For this review, take the finished solid that the model builds, in its own axes (mm). Round coordinates to 2 decimals unless told otherwise and drop trailing zeros. Write each loop counter-clockwise with the first axis right and the second up, starting at its lowest first coordinate (ties: lowest second). Pieces come first, ordered by that corner, then holes. Notation, with made-up numbers: (46.5, 28.25) -> (50.5, 28.25) arc R28 cw to (50.5, 52.25) -> close; hole circle Ø4 at (29, 70). An arc over 180 degrees is marked (long way). Answer in a Markdown table with one row per item.
Autodesk Inventor part; units mm, degrees
ref_plane "Work Plane1" through (-75.4448, 0, 297.9362) normal (-0.2454766, 0, 0.9694025) x (0, -1, 0)
ref_plane "YZ Plane" through (0, 0, 0) normal (1, 0, 0) x (0, 1, 0)
ref_plane "XZ Plane" through (0, 0, 0) normal (0, 1, 0) x (-1, 0, 0)
sketch "Sketch1" plane through (0, 0, 0) normal (0, 1, 0) x (-1, 0, 0)
  arc A0 (307.34, 0) -> (25.3968, 306.2889) centre (0, 0) ccw
  line L0 (0, 0) -> (25.3968, 306.2889) construction
  line L1 (0, 0) -> (307.34, 0) construction
  arc A1 (306.07, 0) -> (25.2919, 305.0232) centre (0, 0) ccw
  line L2 (0, 0) -> (25.2919, 305.0232) construction
  line L3 (0, 0) -> (306.07, 0) construction
  line L4 (25.3968, 306.2889) -> (25.2919, 305.0232)
  line L5 (307.34, 0) -> (306.07, 0)
  dimension "d0" = 307.34
  dimension "d1" = 85.26
  dimension "d2" = 306.07
  dimension "d3" = 85.26
extrude "Extrusion1" add sketch "Sketch1" along normal blind 1625.6
sketch "Sketch2" plane through (0, 0, 0) normal (0, 1, 0) x (-1, 0, 0)
  arc A0 (75.4448, 297.9362) -> (25.3968, 306.2889) centre (0, 0) ccw
  line L0 (0, 0) -> (75.4448, 297.9362) construction
  line L1 (0, 0) -> (25.3968, 306.2889) construction
  arc A1 (123.4855, 281.4413) -> (25.3968, 306.2889) centre (0, 0) ccw
  line L2 (0, 0) -> (123.4855, 281.4413) construction
  line L3 (0, 0) -> (25.3968, 306.2889) construction
  arc A2 (307.34, 0) -> (290.6829, 99.8065) centre (0, 0) ccw
  line L4 (0, 0) -> (290.6829, 99.8065) construction
  line L5 (0, 0) -> (307.34, 0) construction
  dimension "d6" = 9.47
  dimension "d13" = 18.95
  dimension "d14" = 18.95
ref_plane "Work Plane1" through (-75.4448, 0, 297.9362) normal (-0.2454766, 0, 0.9694025) x (0, -1, 0)
sketch "Sketch3" plane through (-75.4448, 0, 297.9362) normal (-0.2454766, 0, 0.9694025) x (0, -1, 0)
  circle A0 centre (-103.1875, 0) radius 25.4
  line L0 (0, 50.567) -> (0, -297.9362)
  line L1 (0, 50.567) -> (-1625.6, 50.567)
  line L2 (-128.5875, 0) -> (-77.7875, 0)
  line L3 (-77.7875, 0) -> (-77.7875, 50.567)
  line L4 (-77.7875, 50.567) -> (-128.5875, 50.567)
  line L5 (-128.5875, 50.567) -> (-128.5875, 0)
  circle A1 centre (-176.2125, 0) radius 25.4
  line L6 (-201.6125, 0) -> (-150.8125, 0)
  line L7 (-150.8125, 0) -> (-150.8125, 50.567)
  line L8 (-150.8125, 50.567) -> (-201.6125, 50.567)
  line L9 (-201.6125, 50.567) -> (-201.6125, 0)
  point P0 (0, 0)
  dimension "d7" = 50.8
  dimension "d9" = 50.8
  dimension "d8" = 103.1875
  dimension "d10" = 176.2125
extrude "Extrusion2" cut sketch "Sketch3" against normal blind 25.4
properties part number "EDM Middle Shield Part 3"
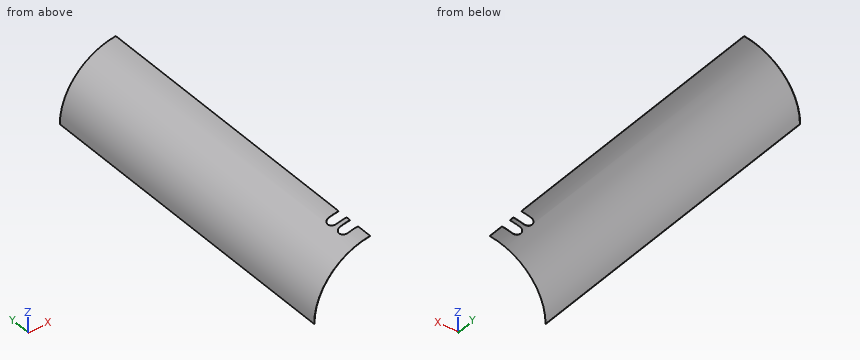
1) For line 1 (Z direction, x = -169.5, y = 1108); line 2 (X direction, y = 515.5, z = 209); line 3 (X direction, y = 601.5, z = 57.5), list the stretches that pass through material, from the lowest coordinate up. Write a range as [from, to].
Solved:
| item | result |
|---|---|
| line 1 | [254.85, 256.37] |
| line 2 | [-225.34, -223.6] |
| line 3 | [-301.91, -300.62] |
2) Consider section A-A on y = 1093.5. State the section outline as (x, z) points, then the cut area to 3 significant figures.
Solved:
| item | result |
|---|---|
| outline | (-307.34, 0) -> (-306.07, 0) arc R306.07 cw to (-25.29, 305.02) -> (-25.4, 306.29) arc R307.34 ccw to start |
| area | 580 mm² |
3) Consider section B-B on x = -173.5. State the section outline as (y, z) points.
Solved:
| item | result |
|---|---|
| outline | (0, 252.14) -> (1625.6, 252.14) -> (1625.6, 253.68) -> (0, 253.68) -> close |
4) Clearance check with flat-ended pins moving along their axes: pin 1 Ø4 at (y, z) = (221, 69.5) entering from +X; pin 2 Ø4 at (y, z) = (575.5, 262.5) entering from -X; pin 3 Ø8 at (y, z) = (618.5, 271.5) entering from +X. State where each tip first meets the part, or that it passes through.
Solved:
| item | result |
|---|---|
| pin 1 | x = -297.6 |
| pin 2 | x = -163.09 |
| pin 3 | x = -133.34 |
